```python
from build123d import *

# Parameters (mm, degrees)
SKETCH1_W                                    = 50.8
SKETCH1_H                                    = 47
SKETCH1_R                                    = 2.1
SKETCH1_H_2                                  = 6
BOSS_EXTRUDE1_DEPTH                          = 6
SKETCH1_5_W                                  = 50.8
SKETCH1_5_H                                  = 6
BOSS_EXTRUDE2_DEPTH                          = 32
CSK_FOR_1_4_FLAT_HEAD_SOCKET_CAP_SCR_2_COUNT = 2
CSK_FOR_1_4_FLAT_HEAD_SOCKET_CAP_SCR_2_PITCH = 30
FILLET1_R                                    = 3
CHAMFER1_SIZE                                = 0.5


with BuildPart() as part:
    # Sketch1 → Boss-Extrude1 (new body)
    with BuildSketch(Plane.XY):
        Rectangle(SKETCH1_W, SKETCH1_H)
        with Locations((7.4, 12.5)):
            Circle(SKETCH1_R, mode=Mode.SUBTRACT)
        with Locations((7.4, -12.5)):
            Circle(SKETCH1_R, mode=Mode.SUBTRACT)
        with Locations((18.4, 0)):
            Circle(SKETCH1_R, mode=Mode.SUBTRACT)
        with Locations((0, -26.5)):
            Rectangle(SKETCH1_W, SKETCH1_H_2)
        Polygon((14.35, 2.33826859), (14.35, -2.33826859), (18.4, -4.67653718), (22.45, -2.33826859), (22.45, 2.33826859), (18.4, 4.67653718), align=None)
        with Locations((18.4, 0)):
            Circle(SKETCH1_R, mode=Mode.SUBTRACT)
        Polygon((3.35, -10.16173141), (3.35, -14.83826859), (7.4, -17.17653718), (11.45, -14.83826859), (11.45, -10.16173141), (7.4, -7.82346282), align=None)
        with Locations((7.4, -12.5)):
            Circle(SKETCH1_R, mode=Mode.SUBTRACT)
        Polygon((11.45, 10.16173141), (11.45, 14.83826859), (7.4, 17.17653718), (3.35, 14.83826859), (3.35, 10.16173141), (7.4, 7.82346282), align=None)
        with Locations((7.4, 12.5)):
            Circle(SKETCH1_R, mode=Mode.SUBTRACT)
    extrude(amount=-BOSS_EXTRUDE1_DEPTH)

    # Sketch1_5 → Boss-Extrude2 (add)
    with BuildSketch(Plane.XY):
        with Locations((0, -26.5)):
            Rectangle(SKETCH1_5_W, SKETCH1_5_H)
    extrude(amount=-BOSS_EXTRUDE2_DEPTH)

    # Sketch4 → CSK for 1_4 Flat Head Socket Cap Screw1 (revolve, cut)
    with BuildSketch(Plane(origin=(-15, -23.5, -20), x_dir=(0, 0, 1), z_dir=(1, 0, 0))):
        Polygon((0, 0), (0, 6), (3.2639, 6), (3.2639, 4.003051983), (6.7437, 0), align=None)
    csk_for_1_4_flat_head_socket_cap_screw1 = revolve(axis=Axis((-15, -17.15, -20), (0, -1, 0)), mode=Mode.SUBTRACT)

    # CSK for 1_4 Flat Head Socket Cap Scr 2: CSK for 1_4 Flat Head Socket Cap Screw1 ×2
    with Locations(*[(i * CSK_FOR_1_4_FLAT_HEAD_SOCKET_CAP_SCR_2_PITCH, 0, 0) for i in range(1, CSK_FOR_1_4_FLAT_HEAD_SOCKET_CAP_SCR_2_COUNT)]):
        add(csk_for_1_4_flat_head_socket_cap_screw1, mode=Mode.SUBTRACT)

    # Fillet1
    fillet1_edges = [part.edges().sort_by_distance(p)[0] for p in [
        (-25.4, 23.5, -3),
        (25.4, 23.5, -3),
        (-25.4, -26.5, -32),
        (25.4, -26.5, -32),
    ]]
    fillet(fillet1_edges, radius=FILLET1_R)

    # Chamfer1
    chamfer1_edges = [part.edges().sort_by_distance(p)[0] for p in [
        (5.3, 12.5, 0),
        (16.3, 0, 0),
        (0, -29.5, 0),
        (16.3, 0, -6),
        (5.3, 12.5, -6),
        (5.3, -12.5, -6),
        (15, -29.5, -23.2639),
        (-15, -29.5, -23.2639),
        (25.4, -29.5, -14.5),
        (25.4, -23.5, -17.5),
        (25.4, -1.5, -6),
        (25.4, -4.5, 0),
        (0, 23.5, 0),
        (-25.4, -4.5, 0),
        (-24.521320344, 22.621320344, 0),
        (24.521320344, 22.621320344, 0),
        (0, 23.5, -6),
        (-25.4, -1.5, -6),
        (-24.521320344, 22.621320344, -6),
        (24.521320344, 22.621320344, -6),
        (-25.4, -29.5, -14.5),
        (-25.4, -23.5, -17.5),
        (0, -23.5, -32),
        (-24.521320344, -23.5, -31.121320344),
        (24.521320344, -23.5, -31.121320344),
        (0, -29.5, -32),
        (-24.521320344, -29.5, -31.121320344),
        (24.521320344, -29.5, -31.121320344),
        (5.3, -12.5, 0),
    ]]
    chamfer(chamfer1_edges, length=CHAMFER1_SIZE)


solid = part.part
```
Source: CAD feature listing. Evaluate the final solid. Frame: model axes, mm. A direction names the side the tool comes from. Give positions to 0.01 mm unless a question says otherwise; leave off trailing zeros. Loops run counter-clockwise (first coordinate to the right, second up) from the corner with the lowest first, then second, coordinate; pieces in that order, holes last. Notation, with made-up numbers: (66.25, 24.25) -> (117.25, 24.25) arc R32 cw to (117.25, 51.25) -> close; hole circle Ø7 at (-19, 77). An arc over 180 degrees is marked (long way). Use a Markdown table: item, result. Add a question column.
(1) Section query A-A (y = 12.5). Output: boundary loops of the cut face in (x, z).
(2) Section query D-D (x = 7.4). Output: boundary loops of the cut face in (y, z), then the cut area to 3 significant figures.
(3) Section query B-B (z = -4.5). Output: boundary loops of the cut face in (x, y).
(4) Pull-direction query (X, two-part tool) for faces 3 (the face through (0, -26, -32)), 4 (the face through (7.127, -10.418, -2.965)), 5 (the face through (24.289, 22.348, -5.858)); classes: +X half, -X half, draft (parallel to the pull), parting line (faces both ways), or undercut.
(5) Access query for faces 1 (the face through (0, -23.5, -19)), 2 (the face through (-25.4, -11, -5)). Directions: +Z, -Z, +X, -X, +Y, -Y. A direction counts if a zero-diameter tool reaches every point of the face in a straight line with its end or side. Return the directions, or none.
(6) Ray query, line 1 (X direction, y = -28.4, z = -20); line 2 (Z direction, x = 15, y = -28); line 3 (Z direction, x = 19, y = -14). Return the intervals inside material, ascending.
(7) Section query C-C (z = -20). Output: boundary loops of the cut face in (x, y), then the cut area to 3 significant figures.
(8) First-contact query: pin 1 Ø5 at (x, y) = (18.4, 0) entering from +Z; pin 2 Ø8 at (x, z) = (-2.5, -12) entering from +Y; pin 3 Ø10 at (x, y) = (20, -16) entering from -Z. Flat tips, straight axial feed; report the tip coordinate or a pass-through.
Checked values:
| question | item | result |
|---|---|---|
| 1 | outline | (-25.4, -5.5) -> (-24.9, -6) -> (4.8, -6) -> (5.3, -5.5) -> (5.3, -0.5) -> (4.8, 0) -> (-24.9, 0) -> (-25.4, -0.5) -> close; (9.5, -5.5) -> (10, -6) -> (24.9, -6) -> (25.4, -5.5) -> (25.4, -0.5) -> (24.9, 0) -> (10, 0) -> (9.5, -0.5) -> close |
| 2 | outline | (-29.5, -31.5) -> (-29, -32) -> (-24, -32) -> (-23.5, -31.5) -> (-23.5, -6) -> (-15.1, -6) -> (-14.6, -5.5) -> (-14.6, -0.5) -> (-15.1, 0) -> (-29, 0) -> (-29.5, -0.5) -> close; (-10.4, -5.5) -> (-9.9, -6) -> (9.9, -6) -> (10.4, -5.5) -> (10.4, -0.5) -> (9.9, 0) -> (-9.9, 0) -> (-10.4, -0.5) -> close; (14.6, -5.5) -> (15.1, -6) -> (23, -6) -> (23.5, -5.5) -> (23.5, -0.5) -> (23, 0) -> (15.1, 0) -> (14.6, -0.5) -> close |
| 2 | area | 422 mm^2 |
| 3 | outline | (-25.4, -29) -> (-24.9, -29.5) -> (24.9, -29.5) -> (25.4, -29) -> (25.4, 20.5) arc R3 ccw to (22.4, 23.5) -> (-22.4, 23.5) arc R3 ccw to (-25.4, 20.5) -> close; hole circle Ø4.2 at (7.4, -12.5); hole circle Ø4.2 at (7.4, 12.5); hole circle Ø4.2 at (18.4, 0) |
| 4 | face 3 | draft |
| 4 | face 4 | undercut |
| 4 | face 5 | +X half |
| 5 | face 1 | -Z, +X, -X, +Y |
| 5 | face 2 | +Z, -Z, -X, +Y, -Y |
| 6 | line 1 | -25.4 to -18.26, -11.74 to 11.74, 18.26 to 25.4 |
| 6 | line 2 | -32 to -23.26, -16.74 to 0 |
| 6 | line 3 | -6 to 0 |
| 7 | outline | (-25.4, -29) -> (-24.9, -29.5) -> (-18.76, -29.5) -> (-18.26, -29) -> (-18.26, -27.5) -> (-21.74, -23.5) -> (-24.9, -23.5) -> (-25.4, -24) -> close; (-11.74, -29) -> (-11.24, -29.5) -> (11.24, -29.5) -> (11.74, -29) -> (11.74, -27.5) -> (8.26, -23.5) -> (-8.26, -23.5) -> (-11.74, -27.5) -> close; (18.26, -29) -> (18.76, -29.5) -> (24.9, -29.5) -> (25.4, -29) -> (25.4, -24) -> (24.9, -23.5) -> (21.74, -23.5) -> (18.26, -27.5) -> close |
| 7 | area | 198 mm^2 |
| 8 | pin 1 | z = -0.1 |
| 8 | pin 2 | y = -23.5 |
| 8 | pin 3 | z = -6 |
